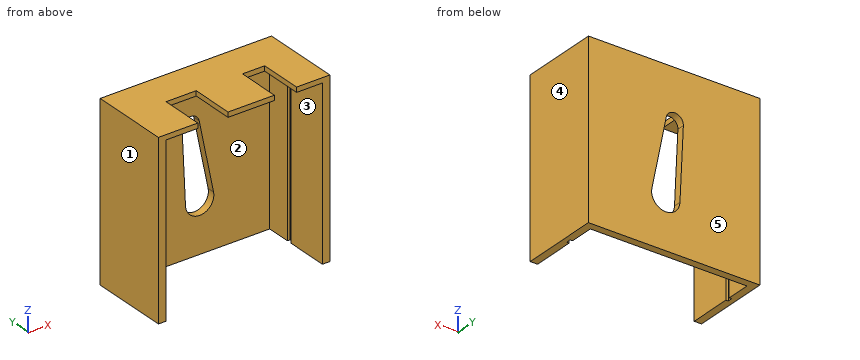
from build123d import *

# Parameters (mm, degrees)
SKETCH2_W           = 35.306
SKETCH2_H           = 71.12
BOSS_EXTRUDE1_DEPTH = 3.048
SKETCH6_W           = 35.306
SKETCH6_H           = 2.032
BOSS_EXTRUDE3_DEPTH = 29.464
SKETCH3_W           = 3.048
SKETCH3_H           = 69.088
BOSS_EXTRUDE2_DEPTH = 29.464
SKETCH4_W           = 1.016
SKETCH4_H           = 1.905
CUT_EXTRUDE1_DEPTH  = 69.088
CUT_EXTRUDE2_DEPTH  = 86.799756293
SKETCH8_W           = 12.446
SKETCH8_H           = 17.78
SKETCH8_W_2         = 9.144
CUT_EXTRUDE3_DEPTH  = 85.691766613


with BuildPart() as part:
    # Sketch2 → Boss-Extrude1 (new body)
    with BuildSketch(Plane(origin=(0, 0, 0), x_dir=(1, 0, 0), z_dir=(0, 1, 0))):
        with Locations((17.653, 35.56)):
            Rectangle(SKETCH2_W, SKETCH2_H)
    boss_extrude1 = extrude(amount=BOSS_EXTRUDE1_DEPTH)

    # Sketch6 → Boss-Extrude3 (add)
    with BuildSketch(Plane.XZ):
        with Locations((17.653, -1.016)):
            Rectangle(SKETCH6_W, SKETCH6_H)
    boss_extrude3 = extrude(amount=BOSS_EXTRUDE3_DEPTH)

    # Sketch3 → Boss-Extrude2 (add)
    with BuildSketch(Plane.XZ):
        with Locations((33.782, -36.576)):
            Rectangle(SKETCH3_W, SKETCH3_H)
    boss_extrude2 = extrude(amount=BOSS_EXTRUDE2_DEPTH)

    # Sketch4 → Cut-Extrude1 (cut)
    with BuildSketch(Plane(origin=(0, 0, -71.12), x_dir=(-1, 0, 0), z_dir=(0, 0, -1))):
        with Locations((-32.766, -10.8585)):
            Rectangle(SKETCH4_W, SKETCH4_H)
    cut_extrude1 = extrude(amount=-CUT_EXTRUDE1_DEPTH, mode=Mode.SUBTRACT)

    # Mirror1: Boss-Extrude1, Boss-Extrude3, Boss-Extrude2, Cut-Extrude1 across plane
    add(boss_extrude1.mirror(Plane(origin=(0, 3.048, 0), x_dir=(0, 0, 1), z_dir=(-1, 0, 0))))
    add(boss_extrude3.mirror(Plane(origin=(0, 3.048, 0), x_dir=(0, 0, 1), z_dir=(-1, 0, 0))))
    add(boss_extrude2.mirror(Plane(origin=(0, 3.048, 0), x_dir=(0, 0, 1), z_dir=(-1, 0, 0))))
    add(cut_extrude1.mirror(Plane(origin=(0, 3.048, 0), x_dir=(0, 0, 1), z_dir=(-1, 0, 0))), mode=Mode.SUBTRACT)

    # Sketch7 → Cut-Extrude2 (cut, through all)
    with BuildSketch(Plane(origin=(0, 3.048, 0), x_dir=(1, 0, 0), z_dir=(0, 1, 0))):
        with BuildLine():
            Line((3.230717937, 20.119567295), (9.153893754, 49.255146271))
            ThreePointArc((9.153893754, 49.255146271), (4.150548543, 56.216269331), (-2.406524046, 50.693996555))
            Line((-2.406524046, 50.693996555), (-3.806058115, 20.995389207))
            ThreePointArc((-3.806058115, 20.995389207), (-0.693203461, 17.299227364), (3.230717937, 20.119567295))
        make_face()
    extrude(amount=-CUT_EXTRUDE2_DEPTH, mode=Mode.SUBTRACT)

    # Sketch8 → Cut-Extrude3 (cut, through all)
    with BuildSketch(Plane.XY):
        with Locations((-12.827, -20.574)):
            Rectangle(SKETCH8_W, SKETCH8_H)
        with Locations((17.018, -20.574)):
            Rectangle(SKETCH8_W_2, SKETCH8_H)
    extrude(amount=-CUT_EXTRUDE3_DEPTH, mode=Mode.SUBTRACT)


solid = part.part
The model under review builds one solid part; all positions refer to its coordinate system, in mm. Face numbers are marked on the shaded views. A direction names the side the tool comes from. Coordinates: 2 decimals unless noted, no trailing zeros. Write each loop counter-clockwise with the first axis right and the second up, starting at its lowest first coordinate (ties: lowest second). Pieces come first, ordered by that corner, then holes. Notation, with made-up numbers: (38, -27.5) -> (81, -27.5) arc R33 ccw to (81, 8.5) -> close; hole circle Ø10 at (-26.75, 36.25). An arc over 180 degrees is marked (long way). Answer in a Markdown table with one row per item.
1. Draft analysis for pull direction X (two halves, no side actions). For the marked faces 3, 4 and 5, state which applies: +X half, -X half, draft (parallel to the pull), parting line (faces both ways), or undercut.
Answers below:
| item | result |
|---|---|
| face 3 | undercut |
| face 4 | +X half |
| face 5 | draft |
2. We need section D-D, the plane y = -9. State the section outline as (x, z) points, and give its area (3 significant figures).
Answers below:
| item | result |
|---|---|
| outline | (-35.31, -71.12) -> (-32.26, -71.12) -> (-32.26, -2.03) -> (32.26, -2.03) -> (32.26, -71.12) -> (35.31, -71.12) -> (35.31, 0) -> (-35.31, 0) -> close |
| area | 565 mm^2 |
3. We need section C-C, the plane x = -10. State the section outline as (y, z) points, and give its area (3 significant figures).
Answers below:
| item | result |
|---|---|
| outline | (-11.68, -2.03) -> (0, -2.03) -> (0, -71.12) -> (3.05, -71.12) -> (3.05, 0) -> (-11.68, 0) -> close |
| area | 241 mm^2 |
4. We need section A-A, the plane y = -15. State the section outline as (x, z) points, and give its area (3 significant figures).
Answers below:
| item | result |
|---|---|
| outline | (-35.31, -71.12) -> (-32.26, -71.12) -> (-32.26, -2.03) -> (-19.05, -2.03) -> (-19.05, 0) -> (-35.31, 0) -> close; (-6.6, -2.03) -> (12.45, -2.03) -> (12.45, 0) -> (-6.6, 0) -> close; (21.59, -2.03) -> (32.26, -2.03) -> (32.26, -71.12) -> (35.31, -71.12) -> (35.31, 0) -> (21.59, 0) -> close |
| area | 521 mm^2 |
5. Wall thickness on probe 1 along X at (y, z) = (-11.5, -41); probe 2 along X at (y, z) = (-14, -27); probe 3 along Y at (x, z) = (9, -66.5): over which ranges is each line inside the solid? List them lowest first. Write a range as [from, to].
Answers below:
| item | result |
|---|---|
| probe 1 | x = [-35.31, -33.27], [33.27, 35.31] |
| probe 2 | x = [-35.31, -32.26], [32.26, 35.31] |
| probe 3 | y = [0, 3.05] |
6. For the marked faces 1 and 2, list the 3-axis set-ups (+Z, -Z, +X, -X, +Y, -Y) from which the entire face can be reached by the end or side of a thin tool; tool diameter is ignored.
Answers below:
| item | result |
|---|---|
| face 1 | +Z, -Z, -X, +Y, -Y |
| face 2 | -Z, -Y |
7. We need section B-B, the plane z = -31.5. State the section outline as (x, y) points, and give its area (3 significant figures).
Answers below:
| item | result |
|---|---|
| outline | (-35.31, -29.46) -> (-32.26, -29.46) -> (-32.26, -11.81) -> (-33.27, -11.81) -> (-33.27, -9.91) -> (-32.26, -9.91) -> (-32.26, 0) -> (-3.31, 0) -> (-3.31, 3.05) -> (-35.31, 3.05) -> close; (5.54, 0) -> (32.26, 0) -> (32.26, -9.91) -> (33.27, -9.91) -> (33.27, -11.81) -> (32.26, -11.81) -> (32.26, -29.46) -> (35.31, -29.46) -> (35.31, 3.05) -> (5.54, 3.05) -> close |
| area | 364 mm^2 |
8. Clearance check with flat-ended pins moving along their axes: pin 1 Ø2 at (x, z) = (-10, -1) entering from -Y; pin 2 Ø1.5 at (x, z) = (2, -19) entering from -Y; pin 3 Ø14.5 at (x, y) = (-12.5, -16.5) entering from -Z. State where each tip first meets the part, or that it passes through.
Answers below:
| item | result |
|---|---|
| pin 1 | stops at y = -11.68 |
| pin 2 | stops at y = 0 |
| pin 3 | stops at z = -2.03 |
